from build123d import *

# Parameters (mm, degrees)
BOSS_EXTRUDE1_DEPTH                                 = 90
SKETCH3_W                                           = 15
SKETCH3_H                                           = 59
CUT_EXTRUDE1_DEPTH                                  = 111.381157812
M6_CLEARANCE_HOLE1_D                                = 6.6
M5_TAPPED_HOLE1_D                                   = 4.2
M5_TAPPED_HOLE1_DEPTH                               = 6
M5_TAPPED_HOLE1_CSINK_D                             = 5.05
M5_TAPPED_HOLE1_CSINK_ANGLE                         = 90
CUT_EXTRUDE2_DEPTH                                  = 112.986606342
M5_TAPPED_HOLE2_D                                   = 4.2
M5_TAPPED_HOLE2_CSINK_D                             = 5.05
M5_TAPPED_HOLE2_CSINK_ANGLE                         = 90
CBORE_FOR_M3_HEX_SOCKET_HEAD_CAP_SCREW1_D           = 3.4
CBORE_FOR_M3_HEX_SOCKET_HEAD_CAP_SCREW1_CBORE_D     = 6.5
CBORE_FOR_M3_HEX_SOCKET_HEAD_CAP_SCREW1_CBORE_DEPTH = 3
CUT_EXTRUDE3_DEPTH                                  = 112.986606342
CUT_EXTRUDE4_DEPTH                                  = 3.2


with BuildPart() as part:
    # Sketch1 → Boss-Extrude1 (new body)
    with BuildSketch(Plane(origin=(0, 0, 0), x_dir=(0, 0, -1), z_dir=(1, 0, 0))):
        Polygon((-60, 0), (-60, -16), (-54, -16), (-54, -6), (-1, -6), (-1, -29), (5, -29), (5, 6), (-1, 6), (-1, 0), align=None)
    extrude(amount=BOSS_EXTRUDE1_DEPTH)

    # Sketch3 → Cut-Extrude1 (cut, through all)
    with BuildSketch(Plane.XZ.offset(16)):
        with Locations((82.5, 30.5)):
            Rectangle(SKETCH3_W, SKETCH3_H)
        with Locations((7.5, 30.5)):
            Rectangle(SKETCH3_W, SKETCH3_H)
    extrude(amount=-CUT_EXTRUDE1_DEPTH, mode=Mode.SUBTRACT)

    # M6 Clearance Hole1 (through all)
    with Locations(Plane.XY.offset(1)):
        with Locations((7.5, -9), (82.5, -9)):
            Hole(M6_CLEARANCE_HOLE1_D / 2)

    # M5 Tapped Hole1
    with Locations(Plane.XY.offset(60)):
        with Locations((45, -11)):
            CounterSinkHole(M5_TAPPED_HOLE1_D / 2, M5_TAPPED_HOLE1_CSINK_D / 2, depth=M5_TAPPED_HOLE1_DEPTH, counter_sink_angle=M5_TAPPED_HOLE1_CSINK_ANGLE)

    # Sketch9 → Cut-Extrude2 (cut, through all)
    with BuildSketch(Plane(origin=(0, 0, 0), x_dir=(1, 0, 0), z_dir=(0, 1, 0))):
        with BuildLine():
            Line((34, -28), (34, -23))
            ThreePointArc((34, -23), (45, -12), (56, -23))
            Line((56, -23), (56, -28))
            ThreePointArc((56, -28), (45, -39), (34, -28))
        make_face()
    extrude(amount=-CUT_EXTRUDE2_DEPTH, mode=Mode.SUBTRACT)

    # M5 Tapped Hole2 (through all)
    with Locations(Plane(origin=(0, 0, 0), x_dir=(-1, 0, 0), z_dir=(0, 1, 0))):
        with Locations((-27, 28), (-63, 28)):
            CounterSinkHole(M5_TAPPED_HOLE2_D / 2, M5_TAPPED_HOLE2_CSINK_D / 2, counter_sink_angle=M5_TAPPED_HOLE2_CSINK_ANGLE)

    # CBORE for M3 Hex Socket Head Cap Screw1 (through all)
    with Locations(Plane(origin=(0, 0, 0), x_dir=(-1, 0, 0), z_dir=(0, 1, 0))):
        with Locations((-29.5, 12.5), (-60.5, 12.5), (-29.5, 43.5), (-60.5, 43.5)):
            CounterBoreHole(CBORE_FOR_M3_HEX_SOCKET_HEAD_CAP_SCREW1_D / 2, CBORE_FOR_M3_HEX_SOCKET_HEAD_CAP_SCREW1_CBORE_D / 2, CBORE_FOR_M3_HEX_SOCKET_HEAD_CAP_SCREW1_CBORE_DEPTH)

    # Sketch15 → Cut-Extrude3 (cut, through all)
    with BuildSketch(Plane(origin=(0, 0, 0), x_dir=(1, 0, 0), z_dir=(0, 1, 0))):
        with BuildLine():
            Line((27.8, -12.5), (27.8, -7.5))
            ThreePointArc((27.8, -7.5), (29.5, -5.8), (31.2, -7.5))
            Line((31.2, -7.5), (31.2, -12.5))
            ThreePointArc((31.2, -12.5), (29.5, -14.2), (27.8, -12.5))
        make_face()
        with BuildLine():
            Line((58.8, -12.5), (58.8, -7.5))
            ThreePointArc((58.8, -7.5), (60.5, -5.8), (62.2, -7.5))
            Line((62.2, -7.5), (62.2, -12.5))
            ThreePointArc((62.2, -12.5), (60.5, -14.2), (58.8, -12.5))
        make_face()
        with BuildLine():
            Line((27.8, -43.5), (27.8, -38.5))
            ThreePointArc((27.8, -38.5), (29.5, -36.8), (31.2, -38.5))
            Line((31.2, -38.5), (31.2, -43.5))
            ThreePointArc((31.2, -43.5), (29.5, -45.2), (27.8, -43.5))
        make_face()
        with BuildLine():
            Line((58.8, -43.5), (58.8, -38.5))
            ThreePointArc((58.8, -38.5), (60.5, -36.8), (62.2, -38.5))
            Line((62.2, -38.5), (62.2, -43.5))
            ThreePointArc((62.2, -43.5), (60.5, -45.2), (58.8, -43.5))
        make_face()
    extrude(amount=-CUT_EXTRUDE3_DEPTH, mode=Mode.SUBTRACT)

    # Sketch16 → Cut-Extrude4 (cut)
    with BuildSketch(Plane(origin=(0, 0, 0), x_dir=(1, 0, 0), z_dir=(0, 1, 0))):
        with BuildLine():
            Line((26.25, -12.5), (26.25, -7.5))
            ThreePointArc((26.25, -7.5), (29.5, -4.25), (32.75, -7.5))
            Line((32.75, -7.5), (32.75, -12.5))
            ThreePointArc((32.75, -12.5), (29.5, -15.75), (26.25, -12.5))
        make_face()
        with BuildLine():
            Line((57.25, -12.5), (57.25, -7.5))
            ThreePointArc((57.25, -7.5), (60.5, -4.25), (63.75, -7.5))
            Line((63.75, -7.5), (63.75, -12.5))
            ThreePointArc((63.75, -12.5), (60.5, -15.75), (57.25, -12.5))
        make_face()
        with BuildLine():
            Line((26.25, -43.5), (26.25, -38.5))
            ThreePointArc((26.25, -38.5), (29.5, -35.25), (32.75, -38.5))
            Line((32.75, -38.5), (32.75, -43.5))
            ThreePointArc((32.75, -43.5), (29.5, -46.75), (26.25, -43.5))
        make_face()
        with BuildLine():
            Line((57.25, -43.5), (57.25, -38.5))
            ThreePointArc((57.25, -38.5), (60.5, -35.25), (63.75, -38.5))
            Line((63.75, -38.5), (63.75, -43.5))
            ThreePointArc((63.75, -43.5), (60.5, -46.75), (57.25, -43.5))
        make_face()
    extrude(amount=-CUT_EXTRUDE4_DEPTH, mode=Mode.SUBTRACT)


solid = part.part
Could you check a few things on this model? Use its own coordinates, in mm. A direction names the side the tool comes from. Coordinates: 2 decimals unless noted, no trailing zeros. Loops run counter-clockwise (first coordinate to the right, second up) from the corner with the lowest first, then second, coordinate; pieces in that order, holes last. Notation, with made-up numbers: (22, -40) -> (46, -40) arc R18 cw to (46, -34) -> close; hole circle Ø3 at (-3, 65.5). An arc over 180 degrees is marked (long way). Answer in a Markdown table with one row per item.
(1) Will these pins go through, and if not, where does the flat tip stop? pin 1 Ø10 at (y, z) = (-24.5, 7) entering from +X; pin 2 Ø8 at (y, z) = (-7, 36) entering from -X; pin 3 Ø3.5 at (y, z) = (-2, 10.5) entering from +X; pin 4 Ø8 at (x, z) = (60.5, 39.5) entering from -Y.
Results found:
| item | result |
|---|---|
| pin 1 | passes through |
| pin 2 | stops at x = 15 |
| pin 3 | stops at x = 75 |
| pin 4 | stops at y = -6 |
(2) If I drill on probe 1 along X at (y, z) = (-3, 28); probe 2 along Y at (x, z) = (7.5, -1.5); probe 3 along Z at (x, y) = (63, -1.85), over which ranges is the centre line in solid material (lowest first)?
Results found:
| item | result |
|---|---|
| probe 1 | x = 15 to 24.9, 29.1 to 34, 56 to 60.9, 65.1 to 75 |
| probe 2 | y = -29 to -12.3, -5.7 to 6 |
| probe 3 | z = -5 to 5.42, 14.58 to 25.9, 30.1 to 36.42, 45.58 to 60 |
(3) Imagine slicing it at A-A (z = 24). List the corners of the cut face in (x, y) for me.
Results found:
| item | result |
|---|---|
| outline | (15, -6) -> (34, -6) -> (34, 0) -> (15, 0) -> close; (56, -6) -> (75, -6) -> (75, 0) -> (56, 0) -> close |
(4) Imagine slicing it at D-D (z = 49.5). List the corners of the cut face in (x, y) for me.
Results found:
| item | result |
|---|---|
| outline | (15, -6) -> (75, -6) -> (75, 0) -> (15, 0) -> close |
(5) Imagine slicing it at C-C (z = 11). List the corners of the cut face in (x, y) for me.
Results found:
| item | result |
|---|---|
| outline | (15, -6) -> (27.8, -6) -> (27.8, -3.2) -> (26.25, -3.2) -> (26.25, 0) -> (15, 0) -> close; (31.2, -6) -> (58.8, -6) -> (58.8, -3.2) -> (57.25, -3.2) -> (57.25, 0) -> (32.75, 0) -> (32.75, -3.2) -> (31.2, -3.2) -> close; (62.2, -6) -> (75, -6) -> (75, 0) -> (63.75, 0) -> (63.75, -3.2) -> (62.2, -3.2) -> close |
(6) Imagine slicing it at B-B (x = 82.5). List the corners of the cut face in (y, z) for me, plus the area to 3 significant figures.
Results found:
| item | result |
|---|---|
| outline | (-29, -5) -> (-12.3, -5) -> (-12.3, 1) -> (-29, 1) -> close; (-5.7, -5) -> (6, -5) -> (6, 1) -> (-5.7, 1) -> close |
| area | 170 mm^2 |
(7) For faces 4 (the face through (75, -5, 37)), 5 (the face through (26.25, -2, 10)), 6 (the face through (60.5, -4.6, 5.8)), 7 (the face through (10.119, -11.008, -2.042)), 8 (the face through (44.6, -13.3, 54)), which set-ups out of +Z, -Z, +X, -X, +Y, -Y let a thin tool reach every point of the face, with its end or its side?
Results found:
| item | result |
|---|---|
| face 4 | +Z, +X, +Y, -Y |
| face 5 | +Y |
| face 6 | +Y, -Y |
| face 7 | +Z, -Z |
| face 8 | +X, -X, -Y |
(8) Thinking about a two-plate mould opening in Z: for faces 1 (the face through (44, -12, -5)), 2 (the face through (29.5, -4.6, 14.2)), 3 (the face through (15, -5, 37)), which applies, released by +Z, released by -Z, zero draft, split by the parting line, or undercut?
Results found:
| item | result |
|---|---|
| face 1 | released by -Z |
| face 2 | undercut |
| face 3 | zero draft |
